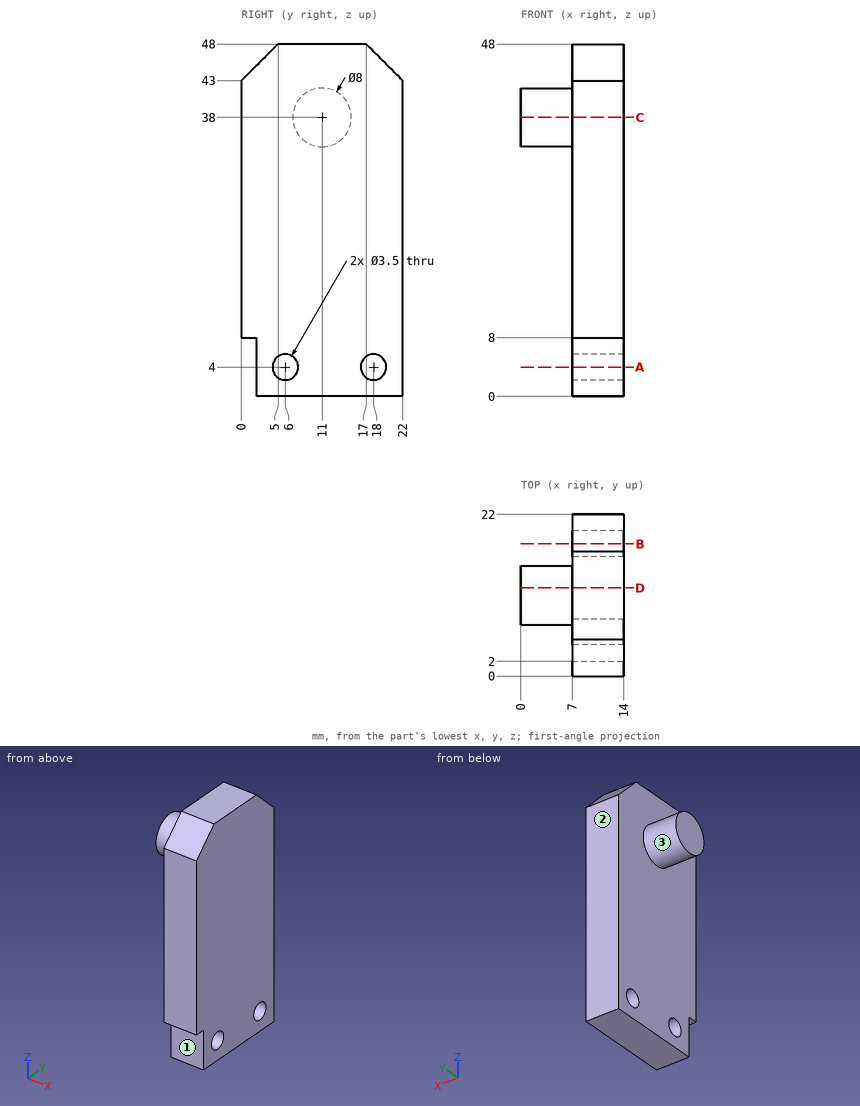
Study the drawing (mm; zero at the part's minimum x, y, z) and answer. A direction names the side the tool comes from. Round coordinates to 2 decimals unless told otherwise and drop trailing zeros. Write each loop counter-clockwise with the first axis right and the second up, starting at its lowest first coordinate (ties: lowest second). Pieces come first, ordered by that corner, then holes. Notation, with made-up numbers: (19, 65.5) - (38, 65.5) arc R9 cw to (38, 74.5) - close; hole circle Ø10 at (19.5, 75). An arc over 180 degrees is marked (long way). Return JSON: item names as keys, results as strings. Group by question number.
Q1. The part is cut by section C-C on z = 38. Write down the section's boundary in (x, y).
Q2. For the marked faces 1, 2 and 3, determine the directions among +Z, -Z, +X, -X, +Y, -Y from which every point of the face is accessible in a straight line to the end or side of a thin tool.
Q3. The part is cut by section D-D on y = 12. Write down the section's boundary in (x, z), then the cut area to 3 significant figures.
Q4. The part is cut by section A-A on z = 4. Write down the section's boundary in (x, y).
Q5. The part is cut by section B-B on y = 18. Write down the section's boundary in (x, z), then the cut area to 4 significant figures.
Q6. Each of these flat-tipped pins is pushed along its axis until it touches: pin 1 Ø3 at (x, z) = (4.5, 18) entering from +Y; pin 2 Ø5.5 at (y, z) = (18, 4) entering from -X; pin 3 Ø7.5 at (x, z) = (9.5, 3.5) entering from -Y; pin 4 Ø3 at (x, y) = (3, 10) entering from +Z. Where does it stop, or does it pass through?
Q7. Find the intervals of material crossed by L1, parallel to Y at x = 12.75, z = 4; L2, parallel to X at y = 18.5, z = 7.5; L3, parallel to Z at x = 12, y = 16.5, in increasing order.
Solved:
{
 "1": {"outline": "(0, 7) - (7, 7) - (7, 0) - (14, 0) - (14, 22) - (7, 22) - (7, 15) - (0, 15) - close"},
 "2": {"face 1": "-Z, +X, -X, -Y", "face 2": "+Z, -Z, +X, -X, +Y", "face 3": "-X"},
 "3": {"outline": "(0, 34.13) - (7, 34.13) - (7, 0) - (14, 0) - (14, 48) - (7, 48) - (7, 41.87) - (0, 41.87) - close", "area": "390 mm²"},
 "4": {"outline": "(7, 2) - (14, 2) - (14, 4.25) - (7, 4.25) - close; (7, 7.75) - (14, 7.75) - (14, 16.25) - (7, 16.25) - close; (7, 19.75) - (14, 19.75) - (14, 22) - (7, 22) - close"},
 "5": {"outline": "(7, 0) - (14, 0) - (14, 2.25) - (7, 2.25) - close; (7, 5.75) - (14, 5.75) - (14, 47) - (7, 47) - close", "area": "304.5 mm²"},
 "6": {"pin 1": "through", "pin 2": "x = 7", "pin 3": "y = 2", "pin 4": "z = 42"},
 "7": {"L1": "2 to 4.25, 7.75 to 16.25, 19.75 to 22", "L2": "7 to 14", "L3": "0 to 3.1, 4.9 to 48"}
}
